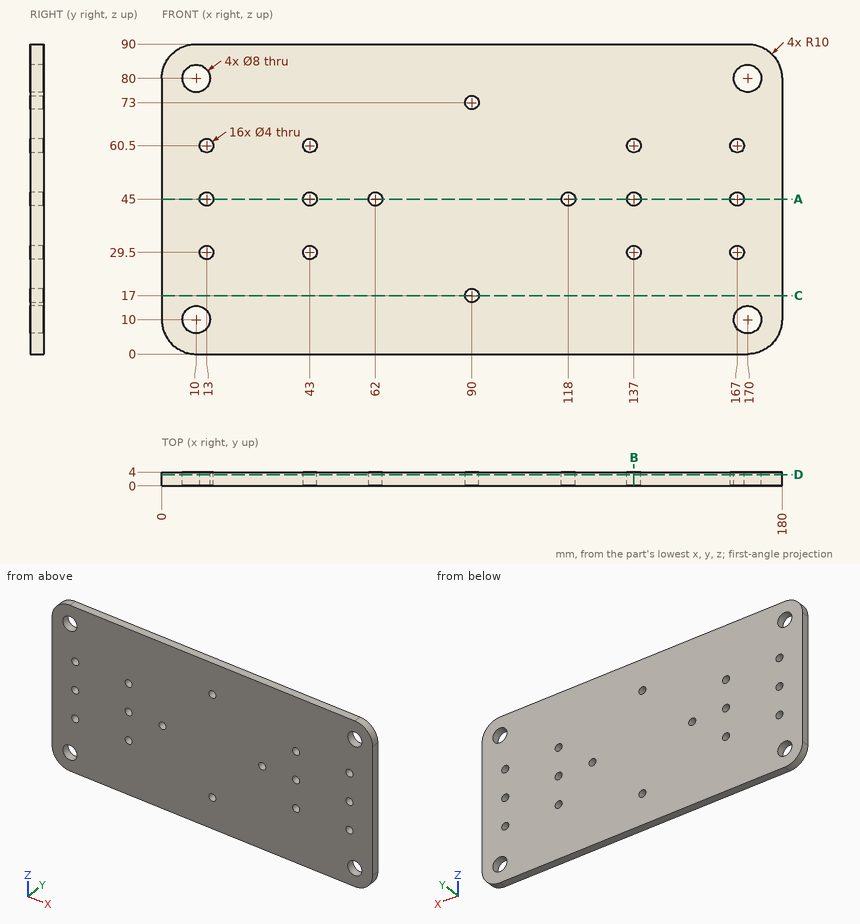
Print and shaded views of the part. All mm, measured from the part's lowest x, y and z. Coordinates: 2 decimals unless noted, no trailing zeros. Loops run counter-clockwise (first coordinate to the right, second up) from the corner with the lowest first, then second, coordinate; pieces in that order, holes last. Notation, with made-up numbers: (40.5, 53) - (98.5, 53) arc R16 ccw to (98.5, 60) - close; hole circle Ø4 at (8.5, 74). An arc over 180 degrees is marked (long way). Write item = value, one per line. Start each with the question number.
Item 1: Flat gauge pins, fed straight in: pin 1 Ø10.5 at (x, z) = (10, 10) entering from -Y; pin 2 Ø2.5 at (x, z) = (43, 45) entering from -Y. Where does each tip first touch, or does it go through?
Item 2: Cut at C-C, the plane z = 17. Give the cut face in (x, y), and give its area (3 significant figures).
Item 3: Wall check: L1, parallel to X at y = 1.55, z = 29.5; L2, parallel to X at y = 3, z = 80; L3, parallel to Z at x = 137, y = 1.85. Give the ranges that are in metal, low to high. Write a range as from..to.
Item 4: Cut at D-D, the plane y = 3.25. State how many separate pieces and enclosed holes the cut face has, and give its area (3 significant figures).
Item 5: Cut at A-A, the plane z = 45. Give the cut face in (x, y).
Item 6: Cut at B-B, the plane x = 137. Give the cut face in (y, z).
The answers:
q1.pin_1 = 0
q1.pin_2 = through
q2.outline = (0, 0) - (88, 0) - (88, 4) - (0, 4) - close; (92, 0) - (180, 0) - (180, 4) - (92, 4) - close
q2.area = 704 mm2
q3.L1 = 0..11, 15..41, 45..135, 139..165, 169..180
q3.L2 = 0..6, 14..166, 174..180
q3.L3 = 0..27.5, 31.5..43, 47..58.5, 62.5..90
q4.separate_pieces = 1
q4.enclosed_holes = 20
q4.area = 15,700 mm2
q5.outline = (0, 0) - (11, 0) - (11, 4) - (0, 4) - close; (15, 0) - (41, 0) - (41, 4) - (15, 4) - close; (45, 0) - (60, 0) - (60, 4) - (45, 4) - close; (64, 0) - (116, 0) - (116, 4) - (64, 4) - close; (120, 0) - (135, 0) - (135, 4) - (120, 4) - close; (139, 0) - (165, 0) - (165, 4) - (139, 4) - close; (169, 0) - (180, 0) - (180, 4) - (169, 4) - close
q6.outline = (0, 0) - (4, 0) - (4, 27.5) - (0, 27.5) - close; (0, 31.5) - (4, 31.5) - (4, 43) - (0, 43) - close; (0, 47) - (4, 47) - (4, 58.5) - (0, 58.5) - close; (0, 62.5) - (4, 62.5) - (4, 90) - (0, 90) - close
